Could you check a few things on this model? Use its own coordinates, in mm. A direction names the side the tool comes from. Coordinates: 2 decimals unless noted, no trailing zeros. Loops run counter-clockwise (first coordinate to the right, second up) from the corner with the lowest first, then second, coordinate; pieces in that order, holes last.
1) If I drill on line 1 along X through (y, z) = (6.5, 4); line 2 along X through (y, z) = (6.5, 3.25); line 3 along X through (y, z) = (7.5, 17.5), over which ranges is the centre line in solid material (lowest first)?
2) Imagine slicing it at C-C on z = 14.5. Please give me the cut outline in (x, y).
3) For faces 1 (the face through (52.22, -0.19, 3.76)), 2 (the face through (11.049, 5, 13)), 3 (the face through (50.1, -1.5, 7.62)), 4 (the face through (22, 10.16, 6)), 5 (the face through (22, 0, 6)), which set-ups out of +Z, -Z, +X, -X, +Y, -Y let a thin tool reach every point of the face, with its end or its side?
4) Imagine slicing it at A-A on x = 5.08. Please give me the cut outline in (y, z).
5) Imagine slicing it at B-B on z = 3.81. Please give me the cut outline in (x, y) (3 decimals).
6) Imagine slicing it at D-D on x = 19.5. Please give me the cut outline in (y, z), plus the area to 3 significant figures.
7) Will these pins go through, and if not, where does the flat tip stop? P1, Ø3, axis at x = 8, y = 6.5, coming from the +Z side; P2, Ø2, axis at x = 14.859, z = 13.589, coming from the +Y side; P3, Ø5, axis at y = 3, z = 14, coming from the +X side; P4, Ø5, axis at y = 4.5, z = 13, coming from the -X side.
8) Thinking about a two-plate mould opening in Z: for faces 6 (the face through (18.669, 5, 13)), 7 (the face through (6, 5, 7.62)), 8 (the face through (14.474, 5.151, 15.325)), which applies, released by +Z, released by -Z, zero draft, split by the parting line, or undercut?
```python
from build123d import *

# Parameters (mm, degrees)
SKETCH1_R           = 1.778
BOSS_EXTRUDE1_DEPTH = 7.62
SKETCH2_R           = 1.778
CUT_EXTRUDE1_DEPTH  = 10.16
SKETCH3_W           = 7.62
SKETCH3_H           = 12.7
SKETCH3_R           = 1.778
BOSS_EXTRUDE2_DEPTH = 10.16
FILLET1_R           = 1.27


with BuildPart() as part:
    # Sketch1 → Boss-Extrude1 (new body)
    with BuildSketch(Plane.XY):
        Polygon((0, 0), (0, 10.16), (43.997363795, 10.16), (81.714794759, -11.61616892), (76.634794759, -20.414987023), (41.275, 0), align=None)
        with Locations((50.578635926, 0.494422029)):
            Circle(SKETCH1_R, mode=Mode.SUBTRACT)
        with Locations((73.675533445, -12.840577971)):
            Circle(SKETCH1_R, mode=Mode.SUBTRACT)
    extrude(amount=BOSS_EXTRUDE1_DEPTH)

    # Sketch2 → Cut-Extrude1 (cut)
    with BuildSketch(Plane(origin=(0, 10.16, 0), x_dir=(1, 0, 0), z_dir=(0, 1, 0))):
        with Locations((5.08, -3.81)):
            Circle(SKETCH2_R)
        with Locations((24.638, -3.81)):
            Circle(SKETCH2_R)
    extrude(amount=-CUT_EXTRUDE1_DEPTH, mode=Mode.SUBTRACT)

    # Sketch3 → Boss-Extrude2 (add)
    with BuildSketch(Plane(origin=(0, 10.16, 0), x_dir=(1, 0, 0), z_dir=(0, 1, 0))):
        with Locations((14.859, -13.97)):
            Rectangle(SKETCH3_W, SKETCH3_H)
        with Locations((14.859, -13.589)):
            Circle(SKETCH3_R, mode=Mode.SUBTRACT)
    extrude(amount=-BOSS_EXTRUDE2_DEPTH)

    # Fillet1
    fillet1_edges = [part.edges().sort_by_distance(p)[0] for p in [
        (0, 0, 3.81),
        (0, 10.16, 3.81),
        (81.714794759, -11.61616892, 3.81),
        (76.634794759, -20.414987023, 3.81),
        (11.049, 5.08, 20.32),
        (18.669, 5.08, 20.32),
    ]]
    fillet(fillet1_edges, radius=FILLET1_R)


solid = part.part
```
Filled in:
1. line 1: x = 0 to 3.31, 6.85 to 22.87, 26.41 to 50.34
1. line 2: x = 0 to 3.39, 6.77 to 22.95, 26.33 to 50.34
1. line 3: x = 11.05 to 18.67
2. outline: (11.05, 0) - (13.33, 0) - (13.33, 10.16) - (11.05, 10.16) - close; (16.39, 0) - (18.67, 0) - (18.67, 10.16) - (16.39, 10.16) - close
3. face 1: +Z, -Z
3. face 2: +Z, -X, +Y, -Y
3. face 3: +Z, +X, +Y, -Y
3. face 4: +Z, -Z, +X, -X, +Y
3. face 5: +Z, -Z, -X, -Y
4. outline: (0, 0) - (10.16, 0) - (10.16, 2.03) - (0, 2.03) - close; (0, 5.59) - (10.16, 5.59) - (10.16, 7.62) - (0, 7.62) - close
5. outline: (0, 1.27) arc R1.27 ccw to (1.27, 0) - (3.302, 0) - (3.302, 10.16) - (1.27, 10.16) arc R1.27 ccw to (0, 8.89) - close; (6.858, 0) - (22.86, 0) - (22.86, 10.16) - (6.858, 10.16) - close; (26.416, 0) - (41.275, 0) - (75.535, -19.78) arc R1.27 ccw to (77.27, -19.315) - (81.08, -12.716) arc R1.27 ccw to (80.615, -10.981) - (43.997, 10.16) - (26.416, 10.16) - close; hole circle Ø3.556 at (50.579, 0.494); hole circle Ø3.556 at (73.676, -12.841)
6. outline: (0, 0) - (10.16, 0) - (10.16, 7.62) - (0, 7.62) - close
6. area: 77.4 mm2
7. P1: stops at z = 7.62
7. P2: passes through
7. P3: stops at x = 18.67
7. P4: stops at x = 11.05
8. face 6: zero draft
8. face 7: released by +Z
8. face 8: undercut
